Can you work these out from the model? Positions are in its coordinate system, mm. A direction names the side the tool comes from. Round coordinates to 2 decimals unless told otherwise and drop trailing zeros. Loops run counter-clockwise (first coordinate to the right, second up) from the corner with the lowest first, then second, coordinate; pieces in that order, holes last.
(1) I want a section at C-C on x = 47. Write out the boundary of the cut face in (y, z), plus the area to 3 significant figures.
(2) If I drill on line 1 along X through (y, z) = (13, -21.5); line 2 along Z through (x, y) = (32, 0); line 3 along Z through (x, y) = (89, 0), over which ranges is the centre line in solid material (lowest first)?
(3) Which directions (+Z, -Z, +X, -X, +Y, -Y) give clear straight access to the entire face, cutting with the end or side of a thin tool? Please do faces 4 (the face through (89.739, -4.769, -21.477)), 5 (the face through (8.218, 0, 0)), 6 (the face through (88.218, -10, -20)).
(4) I want a section at A-A on y = 0. Write out the boundary of the cut face in (x, z).
(5) Thinking about a two-plate mould opening in Z: for faces 1 (the face through (10, -28, -21)), 2 (the face through (11.218, -26, 16)), 3 (the face through (11.218, 0, 0)), which applies, released by +Z, released by -Z, zero draft, split by the parting line, or undercut?
(6) Will these pins go through, and if not, where does the flat tip stop? pin 1 Ø1.5 at (x, z) = (46, -21) entering from +Y; pin 2 Ø4 at (x, y) = (64.5, 5.5) entering from -Z; pin 3 Ø12 at (x, y) = (59.5, 11.5) entering from +Z.
from build123d import *

# Parameters (mm, degrees)
SKETCH2_R           = 27
BOSS_EXTRUDE1_DEPTH = 3


with BuildPart() as part:
    # Sketch1 → Revolve-Thin1 (revolve)
    with BuildSketch(Plane.XY):
        Polygon((8.218422341, 35), (8.218422341, 27), (88.218422341, 27), (88.218422341, 22), (91.218422341, 22), (91.218422341, 30), (11.218422341, 30), (11.218422341, 35), align=None)
    revolve(axis=Axis((0, 0, 0), (1, 0, 0)))

    # Sketch2 → Boss-Extrude1 (add)
    with BuildSketch(Plane.ZY.offset(-8.218422341)):
        Circle(SKETCH2_R)
    extrude(amount=-BOSS_EXTRUDE1_DEPTH)


solid = part.part
Filled sheet:
1. outline: circle Ø60 at (0, 0); hole circle Ø54 at (0, 0)
1. area: 537 mm2
2. line 1: x = 8.22 to 11.22, 88.22 to 91.22
2. line 2: z = -30 to -27, 27 to 30
2. line 3: z = -30 to -22, 22 to 30
3. face 4: +X
3. face 5: +Z, -Z, -X, +Y, -Y
3. face 6: none
4. outline: (8.22, -35) - (11.22, -35) - (11.22, -30) - (91.22, -30) - (91.22, -22) - (88.22, -22) - (88.22, -27) - (11.22, -27) - (11.22, 27) - (88.22, 27) - (88.22, 22) - (91.22, 22) - (91.22, 30) - (11.22, 30) - (11.22, 35) - (8.22, 35) - close
5. face 1: split by the parting line
5. face 2: zero draft
5. face 3: undercut
6. pin 1: stops at y = 22.13
6. pin 2: stops at z = -29.8
6. pin 3: stops at z = 29.49
